Autodesk Inventor part; units mm, degrees
ref_plane "YZ Plane" through (0, 0, 0) normal (1, 0, 0) x (0, 1, 0)
ref_plane "XZ Plane" through (0, 0, 0) normal (0, 1, 0) x (-1, 0, 0)
ref_plane "XY Plane" through (0, 0, 0) normal (0, 0, 1) x (1, 0, 0)
sketch "Sketch1" plane through (0, 0, 0) normal (0, 1, 0) x (-1, 0, 0)
  point P0 (0, 0)
sketch "Sketch2" plane through (0, 0, 0) normal (0, 1, 0) x (-1, 0, 0)
  line L0 (0, 0) -> (0, -7.5)
  line L1 (0, 0) -> (0, 7.5)
  line L2 (0, 7.5) -> (15, 7.5)
  line L3 (0, -7.5) -> (15, -7.5)
  line L4 (15, -7.5) -> (15, 7.5)
  dimension "d0" = 7.5
  dimension "d1" = 7.5
  dimension "d2" = 15
extrude "Extrusion1" add sketch "Sketch2" along normal blind 12
sketch "Sketch3" plane through (-15, 0, 7.5) normal (0, 0, 1) x (1, 0, 0)
  line L0 (0, 0) -> (0, 12)
  circle A0 centre (7.5, 4.5) radius 2.5
  line L1 (0, 12) -> (15, 12)
  point P0 (15, 0)
  dimension "d6" = 5
  dimension "d12" = 7.5
fillet "Fillet1" radius 2 4 edges at (0, 12, -3.75) (-15, 12, 0) (-7.5, 12, 7.5) (-7.5, 12, -7.5)
extrude "Extrusion2" cut sketch "Sketch3" against normal blind 15
fillet "Fillet2" radius 2 6 edges at (-14.4142, 11.4142, 6.9142) (-15, 5, 7.5) (-0.5858, 11.4142, 6.9142) (0, 5, 7.5) (-14.4142, 11.4142, -6.9142) (-15, 5, -7.5)
fillet "Fillet3" radius 2 2 edges at (-0.5858, 11.4142, -6.9142) (0, 5, -7.5)
properties part number "Connector"
Input: part model. Units: mm. Frame: model coordinates. Give positions to 0.01 mm unless a question says otherwise; leave off trailing zeros. Loops run counter-clockwise (first coordinate to the right, second up) from the corner with the lowest first, then second, coordinate; pieces in that order, holes last. Notation, with made-up numbers: (-14.75, 31) - (1.25, 31) arc R13 cw to (1.25, 41) - close; hole circle Ø3 at (40, 33). An arc over 180 degrees is marked (long way). Use CSV: the item, a comma, the result in double quotes. Start each with the question number.
Item 1: Section C-C on z = -4.5. Return loops of the section in (x, y).
Item 2: Section B-B on x = -9. Return loops of the section in (y, z), then the cut area to 3 significant figures.
Item 3: Mould query, pull axis X, two halves, no side actions, for faces 1 (the cylindrical face through (-9.34, 6.19, 0.11)), 2 (the cylindrical face through (-0.57, 4.93, 6.9)), 3 (the flat face through (-7.4, 7.2, 7.5)). Classes: pulls with the +X half, pulls with the -X half, needs draft (parallel to the pull), parting line crosses it, or undercut.
Item 4: Line query: line 1 (Y direction, x = -7.5, z = 4.75); line 2 (Y direction, x = -8, z = -4.25); line 3 (X direction, y = 3.25, z = 6). Output: solid intervals per line, ascending.
Item 5: Section A-A on y = 6. Return loops of the section in (x, z).
Item 6: Contact query for a flat-ended pin moving along its axis: P1, Ø4.5, axis at x = -7.5, y = 4.5, coming from the +Z side. Output: stop coordinate, or through.
Item 7: Section D-D on y = 8.75. Return loops of the section in (x, z).
Ans:
1,outline,"(-15, 0) - (0, 0) - (0, 10) arc R2 ccw to (-2, 12) - (-13, 12) arc R2 ccw to (-15, 10) - close; hole circle Ø5 at (-7.5, 4.5)"
2,outline,"(0, -7.5) - (2.5, -7.5) - (2.5, 7.5) - (0, 7.5) - close; (6.5, -7.5) - (10, -7.5) arc R2 ccw to (12, -5.5) - (12, 5.5) arc R2 ccw to (10, 7.5) - (6.5, 7.5) - close"
2,area,"118 mm2"
3,face 1,"undercut"
3,face 2,"pulls with the +X half"
3,face 3,"needs draft"
4,line 1,"y = 0 to 2, 7 to 12"
4,line 2,"y = 0 to 2.05, 6.95 to 12"
4,line 3,"x = -14.94 to -9.67, -5.33 to -0.06"
5,outline,"(-15, -5.5) arc R2 ccw to (-13, -7.5) - (-9.5, -7.5) - (-9.5, 7.5) - (-13, 7.5) arc R2 ccw to (-15, 5.5) - close; (-5.5, -7.5) - (-2, -7.5) arc R2 ccw to (0, -5.5) - (0, 5.5) arc R2 ccw to (-2, 7.5) - (-5.5, 7.5) - close"
6,P1,"passes through"
7,outline,"(-15, -5.5) arc R2 ccw to (-13, -7.5) - (-2, -7.5) arc R2 ccw to (0, -5.5) - (0, 5.5) arc R2 ccw to (-2, 7.5) - (-13, 7.5) arc R2 ccw to (-15, 5.5) - close"
